Verification items for this drawing (mm, ordinates from the low corner). Give positions to 0.01 mm unless a question says otherwise; leave off trailing zeros. Order: outer loops, then holes, each group sorted by start corner. A loop starts at its lowest first (then second) coordinate and runs counter-clockwise, first axis right, second up. Notation, with made-up numbers: M -11,46.5 L 40,46.5 A25 cw 40,81.5 Z; hole C 86.5,47 d1. An arc over 180 degrees is marked long. Return JSON: item names as keys, results as strings. Group by question number.
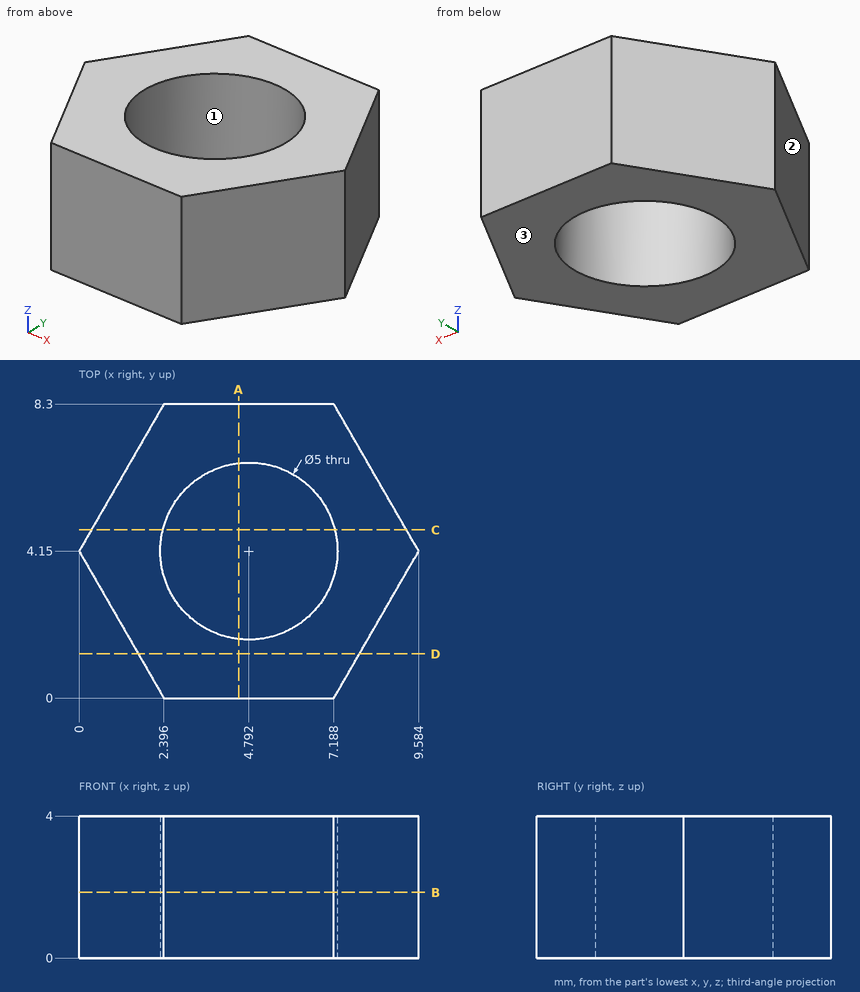
1) Sectioned sample at D-D on y = 1.25. Record the boundary of the cut face in (x, z), then the cut area to 3 significant figures.
2) Sectioned sample at A-A on x = 4.5. Record the boundary of the cut face in (y, z).
3) Sectioned sample at B-B on z = 1.85. Record the boundary of the cut face in (x, y).
4) Material ranges on line 1 along Y through (x, z) = (3, 2.35); line 2 along X through (y, z) = (4, 0.4); line 3 along Y through (x, z) = (5.75, 3.45), recorded low to high.
5) Sectioned sample at C-C on y = 4.75. Record the boundary of the cut face in (x, z), then the cut area to 4 significant figures.
6) Release check for a two-part mould opening along X. For the marked faces 1, 2 and 3 record: released by +X, released by -X, zero draft, split by the parting line, or undercut.
7) Depth check by flat-ended pin: P1, Ø2, axis at y = 6, z = 3.5, coming from the +X side; P2, Ø1.5, axis at y = 6.5, z = 3, coming from the +X side. Enter the tip coordinate at first touch or a pass-through.
Reply:
{
 "1": {"outline": "M 1.67,0 L 7.91,0 L 7.91,4 L 1.67,4 Z", "area": "24.9 mm^2"},
 "2": {"outline": "M 0,0 L 1.67,0 L 1.67,4 L 0,4 Z; M 6.63,0 L 8.3,0 L 8.3,4 L 6.63,4 Z"},
 "3": {"outline": "M 0,4.15 L 2.4,0 L 7.19,0 L 9.58,4.15 L 7.19,8.3 L 2.4,8.3 Z; hole C 4.79,4.15 d5"},
 "4": {"line 1": "0 to 2.41, 5.89 to 8.3", "line 2": "0.09 to 2.3, 7.29 to 9.5", "line 3": "0 to 1.84, 6.46 to 8.3"},
 "5": {"outline": "M 0.35,0 L 2.37,0 L 2.37,4 L 0.35,4 Z; M 7.22,0 L 9.24,0 L 9.24,4 L 7.22,4 Z", "area": "16.15 mm^2"},
 "6": {"face 1": "undercut", "face 2": "released by -X", "face 3": "zero draft"},
 "7": {"P1": "x = 9.09", "P2": "x = 8.66"}
}
